Part model, mm, in its own coordinate system. Coordinates: 2 decimals unless noted, no trailing zeros. Write each loop counter-clockwise with the first axis right and the second up, starting at its lowest first coordinate (ties: lowest second). Pieces come first, ordered by that corner, then holes. Notation, with made-up numbers: (53.25, 84.25) -> (90.25, 84.25) arc R29 ccw to (90.25, 108.25) -> close; hole circle Ø11 at (-32.75, -6.75). An arc over 180 degrees is marked (long way). Write item = value, one per line.
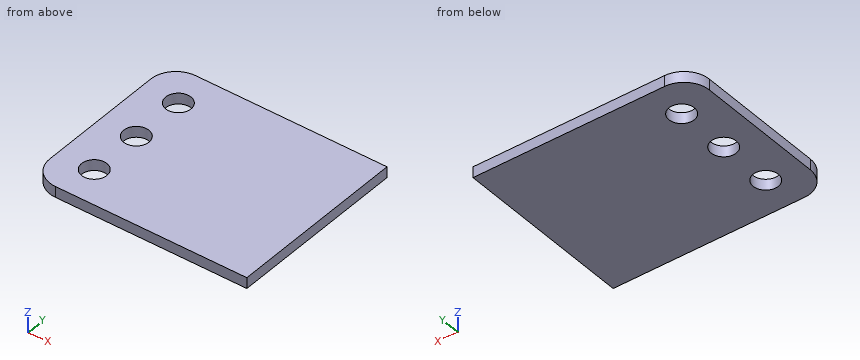
from build123d import *

# Parameters (mm, degrees)
ESQUISSE1_W             = 60
ESQUISSE1_H             = 50
BOSS_EXTRU_1_DEPTH      = 3
ESQUISSE2_R             = 3.5
ENL_V_MAT_EXTRU_1_DEPTH = 3
CONG_1_R                = 7


with BuildPart() as part:
    # Esquisse1 → Boss.-Extru.1 (new body)
    with BuildSketch(Plane.XY):
        with Locations((30, 25)):
            Rectangle(ESQUISSE1_W, ESQUISSE1_H)
    extrude(amount=BOSS_EXTRU_1_DEPTH)

    # Esquisse2 → Enlèv. mat.-Extru.1 (cut)
    with BuildSketch(Plane.XY.offset(3)):
        with Locations((10, 10)):
            Circle(ESQUISSE2_R)
        with Locations((10, 25)):
            Circle(ESQUISSE2_R)
        with Locations((10, 40)):
            Circle(ESQUISSE2_R)
    extrude(amount=-ENL_V_MAT_EXTRU_1_DEPTH, mode=Mode.SUBTRACT)

    # Congé1
    cong_1_edges = [part.edges().sort_by_distance(p)[0] for p in [
        (0, 50, 1.5),
        (0, 0, 1.5),
    ]]
    fillet(cong_1_edges, radius=CONG_1_R)


solid = part.part
Q1. Saw through at D-D on y = 22.5. Give the cut face in (x, z).
Model answer:
outline = (0, 0) -> (7.55, 0) -> (7.55, 3) -> (0, 3) -> close; (12.45, 0) -> (60, 0) -> (60, 3) -> (12.45, 3) -> close
Q2. Pin check, flat tips, straight feed: pin 1 (8 mm diameter, centred on x = 10, y = 25, fed in from -Z); pin 2 (5.5 mm diameter, centred on x = 10, y = 10, fed in from -Z). Stop position of each tip, or through.
Model answer:
pin_1 = 0
pin_2 = through
Q3. Saw through at B-B on x = 10. Give the cut face in (y, z).
Model answer:
outline = (0, 0) -> (6.5, 0) -> (6.5, 3) -> (0, 3) -> close; (13.5, 0) -> (21.5, 0) -> (21.5, 3) -> (13.5, 3) -> close; (28.5, 0) -> (36.5, 0) -> (36.5, 3) -> (28.5, 3) -> close; (43.5, 0) -> (50, 0) -> (50, 3) -> (43.5, 3) -> close
Q4. Probe line 1 (Y direction, x = 10, z = 0.95); line 2 (Y direction, x = 7, z = 0.75); line 3 (X direction, y = 27, z = 2.3). List the from-to ranges inside material, lowest first. Write a range as from..to.
Model answer:
line_1 = 0..6.5, 13.5..21.5, 28.5..36.5, 43.5..50
line_2 = 0..8.2, 11.8..23.2, 26.8..38.2, 41.8..50
line_3 = 0..7.13, 12.87..60
Q5. Saw through at C-C on y = 40. Give the cut face in (x, z).
Model answer:
outline = (0, 0) -> (6.5, 0) -> (6.5, 3) -> (0, 3) -> close; (13.5, 0) -> (60, 0) -> (60, 3) -> (13.5, 3) -> close
Q6. Saw through at A-A on z = 1.5. Give the cut face in (x, y), and give its area (3 significant figures).
Model answer:
outline = (0, 7) arc R7 ccw to (7, 0) -> (60, 0) -> (60, 50) -> (7, 50) arc R7 ccw to (0, 43) -> close; hole circle Ø7 at (10, 10); hole circle Ø7 at (10, 25); hole circle Ø7 at (10, 40)
area = 2,860 mm²
